Work out the finished part from the listing and answer in its coordinate system (mm). Give positions to 0.01 mm unless a question says otherwise; leave off trailing zeros. Order: outer loops, then holes, each group sorted by start corner. A loop starts at its lowest first (then second) coordinate and runs counter-clockwise, first axis right, second up. Notation, with made-up numbers: (37.25, 63) - (66.25, 63) arc R31 ccw to (66.25, 93) - close; hole circle Ø9 at (-40, 61). An arc over 180 degrees is marked (long way). Put each result on its own line as item: value.
```python
from build123d import *

# Parameters (mm, degrees)
SKETCH1_W           = 38.5
SKETCH1_H           = 8.5
BOSS_EXTRUDE1_DEPTH = 2
SKETCH2_W           = 0.8
SKETCH2_H           = 6.15
BOSS_EXTRUDE2_DEPTH = 1.7
SKETCH3_W           = 32.5
SKETCH3_H           = 4.5
CUT_EXTRUDE1_DEPTH  = 21.057791504


with BuildPart() as part:
    # Sketch1 → Boss-Extrude1 (new body)
    with BuildSketch(Plane.XY):
        Rectangle(SKETCH1_W, SKETCH1_H)
    extrude(amount=BOSS_EXTRUDE1_DEPTH)

    # Sketch2 → Boss-Extrude2 (add)
    with BuildSketch(Plane(origin=(0, 0, 0), x_dir=(-1, 0, 0), z_dir=(0, 0, -1))):
        with Locations((-18, -0.325)):
            Rectangle(SKETCH2_W, SKETCH2_H)
    boss_extrude2 = extrude(amount=BOSS_EXTRUDE2_DEPTH)

    # Mirror1: Boss-Extrude2 across plane
    add(boss_extrude2.mirror(Plane(origin=(0, 0, 0), x_dir=(0, 0, 1), z_dir=(1, 0, 0))))

    # Sketch3 → Cut-Extrude1 (cut, through all)
    with BuildSketch(Plane.XY.offset(2)):
        with Locations((0, 2)):
            Rectangle(SKETCH3_W, SKETCH3_H)
    extrude(amount=-CUT_EXTRUDE1_DEPTH, mode=Mode.SUBTRACT)


solid = part.part
```
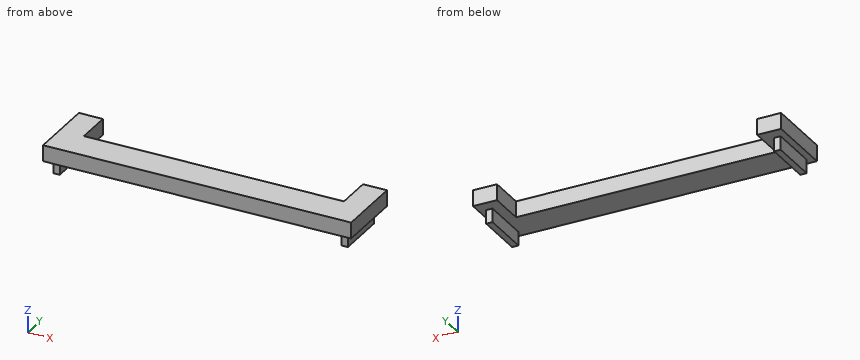
(1) Section A-A, the plane y = 2 is taken. Write down the section's boundary in (x, z), then the cut area to 3 significant figures.
Geometry check:
outline: (-19.25, 0) - (-18.4, 0) - (-18.4, -1.7) - (-17.6, -1.7) - (-17.6, 0) - (-16.25, 0) - (-16.25, 2) - (-19.25, 2) - close; (16.25, 0) - (17.6, 0) - (17.6, -1.7) - (18.4, -1.7) - (18.4, 0) - (19.25, 0) - (19.25, 2) - (16.25, 2) - close
area: 14.7 mm²
(2) Section C-C, the plane z = -1.25 is taken. Write down the section's boundary in (x, y).
Geometry check:
outline: (-18.4, -3.4) - (-17.6, -3.4) - (-17.6, 2.75) - (-18.4, 2.75) - close; (17.6, -3.4) - (18.4, -3.4) - (18.4, 2.75) - (17.6, 2.75) - close
(3) Straight lines are drawn through the part: line 1 (X direction, y = 0, z = -1.05); line 2 (X direction, y = 3.5, z = 0.8); line 3 (Y direction, x = -5.5, z = 0.45). For each, find the intervals that lie inside material, in ascending order.
Geometry check:
line 1: x = -18.4 to -17.6, 17.6 to 18.4
line 2: x = -19.25 to -16.25, 16.25 to 19.25
line 3: y = -4.25 to -0.25
(4) Given pin 1 (2 mm diameter, centred on x = 9, y = 0.5, fed in from -Z); pin 2 (1.4 mm diameter, centred on y = 0.5, z = -0.5, fed in from +X); pin 3 (1.6 mm diameter, centred on x = -6, z = 0.5, fed in from +Y); pin 4 (0.9 mm diameter, centred on x = 18, z = -0.5, fed in from -Y), each flat-ended and moving along its own axis, determine where each tip first touches the part or whether it passes through.
Geometry check:
pin 1: stops at z = 0
pin 2: stops at x = 19.25
pin 3: stops at y = -0.25
pin 4: stops at y = -3.4
(5) Section D-D, the plane y = -2.25 is taken. Write down the section's boundary in (x, z).
Geometry check:
outline: (-19.25, 0) - (-18.4, 0) - (-18.4, -1.7) - (-17.6, -1.7) - (-17.6, 0) - (17.6, 0) - (17.6, -1.7) - (18.4, -1.7) - (18.4, 0) - (19.25, 0) - (19.25, 2) - (-19.25, 2) - close
(6) Section B-B, the plane z = 0.6 is taken. Write down the section's boundary in (x, y).
Geometry check:
outline: (-19.25, -4.25) - (19.25, -4.25) - (19.25, 4.25) - (16.25, 4.25) - (16.25, -0.25) - (-16.25, -0.25) - (-16.25, 4.25) - (-19.25, 4.25) - close
